Geometry check sheet. Reference: the model listing, model coordinates, mm. Face numbers are marked on the shaded views. A direction names the side the tool comes from. Coordinates: 2 decimals unless noted, no trailing zeros. Order: outer loops, then holes, each group sorted by start corner. A loop starts at its lowest first (then second) coordinate and runs counter-clockwise, first axis right, second up. Notation, with made-up numbers: (23, -13) - (29, -13) arc R33 cw to (29, 15) - close; hole circle Ø10 at (-6, 88.5). An arc over 180 degrees is marked (long way). Use CSV: the item, a comma, the result in double quotes. Start each with the question number.
1) Sectioned sample at D-D, the plane z = -8. Record the cut outline in (x, y).
2) Depth check by flat-ended pin: P1, Ø1.5, axis at x = -30, y = 3, coming from the +Z side; P2, Ø16.5, axis at x = -18.5, z = -4.5, coming from the -Y side; P3, Ø5, axis at x = 14, y = -152.15, coming from the -Z side. Enter the tip coordinate at first touch or a pass-through.
3) Thickness scan on probe 1 along Y at (x, z) = (28, -17); probe 2 along X at (y, z) = (-152.15, 51.15); probe 3 along Y at (x, z) = (14, 52.15). Record the ranges inside material, lowest first. Write a range as [from, to].
4) Draft check along X on the marked faces 1, 2, 3 and 4. Enter one of: released by +X, released by -X, zero draft, split by the parting line, or undercut.
5) Sectioned sample at C-C, the plane y = -180.15. Record the cut outline in (x, z), and give its area (3 significant figures).
6) Sectioned sample at B-B, the plane y = 10. Record the cut outline in (x, z), and give its area (3 significant figures).
7) Sectioned sample at A-A, the plane x = 28. Record the cut outline in (y, z), and give its area (3 significant figures).
8) Tool access check on the marked faces 5, 6 and 7. Record the directions out of +Z, -Z, +X, -X, +Y, -Y that give a thin tool (end or side, any length) a straight path to the whole face; none if there is none.
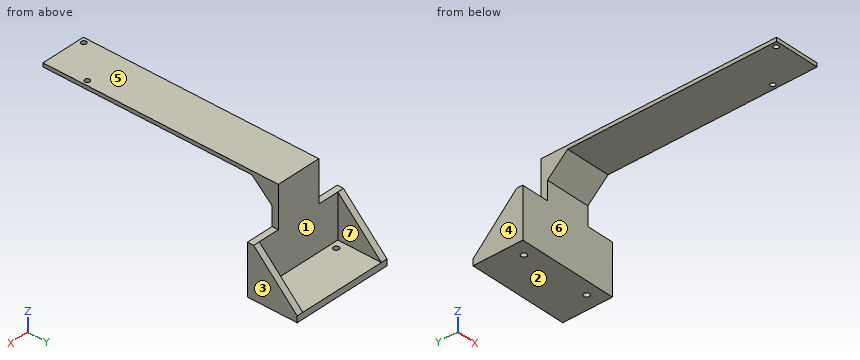
from build123d import *

# Parameters (mm, degrees)
SKETCH1_W           = 80
SKETCH1_H           = 40
BOSS_EXTRUDE1_DEPTH = 5
SKETCH2_W           = 80
SKETCH2_H           = 5
BOSS_EXTRUDE2_DEPTH = 35
BOSS_EXTRUDE3_DEPTH = 5
BOSS_EXTRUDE4_DEPTH = 5
SKETCH6_R           = 2.2
CUT_EXTRUDE2_DEPTH  = 6
SKETCH7_W           = 36
SKETCH7_H           = 5
BOSS_EXTRUDE5_DEPTH = 33
SKETCH8_W           = 36
SKETCH8_H           = 3
BOSS_EXTRUDE6_DEPTH = 184.15
BOSS_EXTRUDE7_DEPTH = 36
SKETCH10_R          = 2
CUT_EXTRUDE3_DEPTH  = 3


with BuildPart() as part:
    # Sketch1 → Boss-Extrude1 (new body)
    with BuildSketch(Plane(origin=(0, 0, 0), x_dir=(1, 0, 0), z_dir=(0, 1, 0))):
        Rectangle(SKETCH1_W, SKETCH1_H)
    extrude(amount=BOSS_EXTRUDE1_DEPTH)

    # Sketch2 → Boss-Extrude2 (add)
    with BuildSketch(Plane(origin=(0, 5, 0), x_dir=(1, 0, 0), z_dir=(0, 1, 0))):
        with Locations((0, 17.5)):
            Rectangle(SKETCH2_W, SKETCH2_H)
    extrude(amount=BOSS_EXTRUDE2_DEPTH)

    # Sketch3 → Boss-Extrude3 (add)
    with BuildSketch(Plane.ZY.offset(40)):
        Polygon((-15, 40), (20, 5), (-15, 5), align=None)
    extrude(amount=-BOSS_EXTRUDE3_DEPTH)

    # Sketch4 → Boss-Extrude4 (add)
    with BuildSketch(Plane(origin=(40, 0, 0), x_dir=(0, 0, -1), z_dir=(1, 0, 0))):
        Polygon((15, 40), (-20, 5), (15, 5), align=None)
    extrude(amount=-BOSS_EXTRUDE4_DEPTH)

    # Sketch6 → Cut-Extrude2 (cut, through all)
    with BuildSketch(Plane.XY.offset(-15)):
        with Locations((-28, 10)):
            Circle(SKETCH6_R)
        with Locations((28, 10)):
            Circle(SKETCH6_R)
    extrude(amount=-CUT_EXTRUDE2_DEPTH, mode=Mode.SUBTRACT)

    # Sketch7 → Boss-Extrude5 (add)
    with BuildSketch(Plane.XY.offset(20)):
        with Locations((0, 2.5)):
            Rectangle(SKETCH7_W, SKETCH7_H)
    extrude(amount=BOSS_EXTRUDE5_DEPTH)

    # Sketch8 → Boss-Extrude6 (add)
    with BuildSketch(Plane.XZ):
        with Locations((0, 51.5)):
            Rectangle(SKETCH8_W, SKETCH8_H)
    extrude(amount=BOSS_EXTRUDE6_DEPTH)

    # Sketch9 → Boss-Extrude7 (add)
    with BuildSketch(Plane.ZY.offset(18)):
        Polygon((35, 0), (50, -16.245521775), (50, 0), align=None)
    extrude(amount=-BOSS_EXTRUDE7_DEPTH)

    # Sketch10 → Cut-Extrude3 (cut)
    with BuildSketch(Plane.XY.offset(53)):
        with Locations((14, -152.15)):
            Circle(SKETCH10_R)
        with Locations((-14, -180.15)):
            Circle(SKETCH10_R)
    extrude(amount=-CUT_EXTRUDE3_DEPTH, mode=Mode.SUBTRACT)


solid = part.part
Evaluation:
1,outline,"(-40, 0) - (40, 0) - (40, 33) - (35, 33) - (35, 5) - (-35, 5) - (-35, 33) - (-40, 33) - close"
2,P1,"z = 20"
2,P2,"y = 0"
2,P3,"z = 50"
3,probe 1,"[0, 7.8], [12.2, 40]"
3,probe 2,"[-18, 12], [16, 18]"
3,probe 3,"[-184.15, -154.15], [-150.15, 5]"
4,face 1,"undercut"
4,face 2,"zero draft"
4,face 3,"released by +X"
4,face 4,"released by -X"
5,outline,"(-18, 50) - (-16, 50) - (-16, 53) - (-18, 53) - close; (-12, 50) - (18, 50) - (18, 53) - (-12, 53) - close"
5,area,"96.0 mm²"
6,outline,"(-40, -20) - (-30.2, -20) - (-30.2, -15) - (-35, -15) - (-35, 15) - (-40, 15) - close; (-25.8, -20) - (25.8, -20) - (25.8, -15) - (-25.8, -15) - close; (30.2, -20) - (40, -20) - (40, 15) - (35, 15) - (35, -15) - (30.2, -15) - close"
6,area,"656 mm²"
7,outline,"(0, -20) - (7.8, -20) - (7.8, -15) - (5, -15) - (5, 20) - (0, 20) - close; (12.2, -20) - (40, -20) - (40, -15) - (12.2, -15) - close"
7,area,"353 mm²"
8,face 5,"+Z, +X, -X, +Y, -Y"
8,face 6,"-Z, +X, -X, -Y"
8,face 7,"+Z, +Y"
